Here's how the part is built. I have some questions about the finished solid (model axes, mm). A direction names the side the tool comes from. Round coordinates to 2 decimals unless told otherwise and drop trailing zeros. Order: outer loops, then holes, each group sorted by start corner. A loop starts at its lowest first (then second) coordinate and runs counter-clockwise, first axis right, second up. Notation, with made-up numbers: (5.25, 31) -> (49.25, 31) arc R15 ccw to (49.25, 43) -> close; hole circle Ø8 at (86, -18). An arc over 180 degrees is marked (long way). Answer in a Markdown table with one row per item.
```python
from build123d import *

# Parameters (mm, degrees)
SKETCH1_R           = 1
SKETCH1_W           = 24
SKETCH1_H           = 13
BOSS_EXTRUDE1_DEPTH = 3


with BuildPart() as part:
    # Sketch1 → Boss-Extrude1 (new body)
    with BuildSketch(Plane(origin=(0, 0, 0), x_dir=(1, 0, 0), z_dir=(0, 1, 0))):
        Polygon((-18, -10), (18, -10), (18, 10), (18, 13), (14, 13), (14, 10), (10, 10), (10, 13), (6, 13), (6, 10), (2, 10), (2, 13), (-2, 13), (-2, 10), (-6, 10), (-6, 13), (-10, 13), (-10, 10), (-14, 10), (-14, 13), (-18, 13), (-18, 10), align=None)
        with Locations(Location((-13.625, 0, 0), (0, 0, 270))):
            Circle(SKETCH1_R, mode=Mode.SUBTRACT)
        with Locations(Location((13.625, 0, 0), (0, 0, 90))):
            Circle(SKETCH1_R, mode=Mode.SUBTRACT)
        Rectangle(SKETCH1_W, SKETCH1_H, mode=Mode.SUBTRACT)
    extrude(amount=BOSS_EXTRUDE1_DEPTH)


solid = part.part
```
1. Suppose I cut it at A-A on z = -4.5. Write out the boundary of the cut face in (x, y).
Numbers:
| item | result |
|---|---|
| outline | (-18, 0) -> (-12, 0) -> (-12, 3) -> (-18, 3) -> close; (12, 0) -> (18, 0) -> (18, 3) -> (12, 3) -> close |
2. For pin 1 Ø0.9 at (x, y) = (4, 2) entering from -Z, with a flat end and sliding along its axis, tell me the tip position at first contact or that it passes through.
Numbers:
| item | result |
|---|---|
| pin 1 | stops at z = -10 |
3. Suppose I cut it at B-B on z = 0. Write out the boundary of the cut face in (x, y) (3 decimals), then the cut area to 3 significant figures.
Numbers:
| item | result |
|---|---|
| outline | (-18, 0) -> (-14.625, 0) -> (-14.625, 3) -> (-18, 3) -> close; (-12.625, 0) -> (-12, 0) -> (-12, 3) -> (-12.625, 3) -> close; (12, 0) -> (12.625, 0) -> (12.625, 3) -> (12, 3) -> close; (14.625, 0) -> (18, 0) -> (18, 3) -> (14.625, 3) -> close |
| area | 24.0 mm2 |
4. We'd pull the mould along X, two halves only. Please class faces 4 (the face through (18, 1, -1)), 5 (the face through (0, 1, 6.5)), 6 (the face through (8, 1, -13)): released by +X, released by -X, zero draft, split by the parting line, or undercut.
Numbers:
| item | result |
|---|---|
| face 4 | released by +X |
| face 5 | undercut |
| face 6 | zero draft |
5. Please list where these lines run through material, in increasing order: line 1 along X through (y, z) = (1.3, -10.5); line 2 along X through (y, z) = (1.8, 0) (3 decimals); line 3 along Z through (x, y) = (0.5, 0.4).
Numbers:
| item | result |
|---|---|
| line 1 | x = -18 to -14, -10 to -6, -2 to 2, 6 to 10, 14 to 18 |
| line 2 | x = -18 to -14.625, -12.625 to -12, 12 to 12.625, 14.625 to 18 |
| line 3 | z = -13 to -6.5, 6.5 to 10 |
6. For faces 1 (the face through (-8, 1, -13)), 2 (the face through (12, 1, 0)), 3 (the face through (10, 1, -11)), which set-ups out of +Z, -Z, +X, -X, +Y, -Y let a thin tool reach every point of the face, with its end or its side?
Numbers:
| item | result |
|---|---|
| face 1 | -Z, +X, -X, +Y, -Y |
| face 2 | +Y, -Y |
| face 3 | -Z, +Y, -Y |
7. Suppose I cut it at C-C on x = 11.5. Write out the boundary of the cut face in (y, z).
Numbers:
| item | result |
|---|---|
| outline | (0, -10) -> (3, -10) -> (3, -6.5) -> (0, -6.5) -> close; (0, 6.5) -> (3, 6.5) -> (3, 10) -> (0, 10) -> close |
8. Suppose I cut it at D-D on y = 0.85. Write out the boundary of the cut face in (x, z) (3 decimals).
Numbers:
| item | result |
|---|---|
| outline | (-18, -13) -> (-14, -13) -> (-14, -10) -> (-10, -10) -> (-10, -13) -> (-6, -13) -> (-6, -10) -> (-2, -10) -> (-2, -13) -> (2, -13) -> (2, -10) -> (6, -10) -> (6, -13) -> (10, -13) -> (10, -10) -> (14, -10) -> (14, -13) -> (18, -13) -> (18, 10) -> (-18, 10) -> close; hole circle Ø2 at (-13.625, 0); hole (-12, -6.5) -> (12, -6.5) -> (12, 6.5) -> (-12, 6.5) -> close; hole circle Ø2 at (13.625, 0) |
